The listing builds one solid part. Answer for the finished solid, in the listing's coordinates (mm). Face numbers are marked on the shaded views. A direction names the side the tool comes from. Coordinates: 2 decimals unless noted, no trailing zeros. Write each loop counter-clockwise with the first axis right and the second up, starting at its lowest first coordinate (ties: lowest second). Pieces come first, ordered by that corner, then holes. Notation, with made-up numbers: M 10.25,-30 L 50.25,-30 A21 ccw 50.25,-16 Z; hole C 38.25,-3.75 d5. An arc over 180 degrees is marked long. Answer as CSV lines item,"result". Start each with the question number.
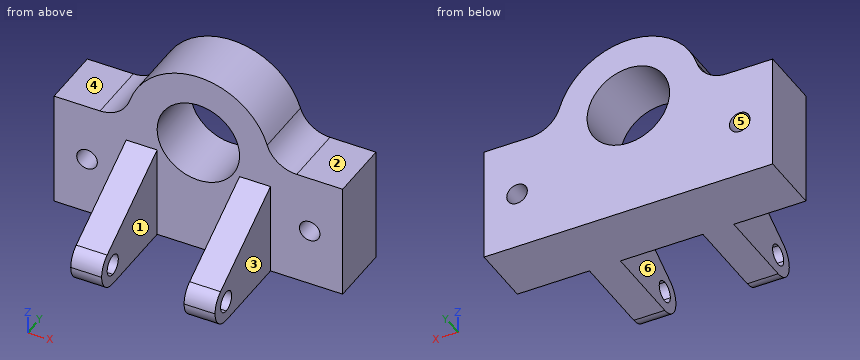
```python
from build123d import *

# Parameters (mm, degrees)
F1_DEPTH = 30
F2_R     = 15
F3_R     = 5
F4_DEPTH = 72
F6_DEPTH = 60
F8_DEPTH = 51.3


with BuildPart() as f1:
    # F0 (on Front) → F1 (new body)
    with BuildSketch(Plane.XZ):
        with BuildLine():
            Line((70, -28), (70, 28))
            Line((70, 28), (35, 28))
            ThreePointArc((35, 28), (0, -7), (-35, 28))
            Line((-35, 28), (-70, 28))
            Line((-70, 28), (-70, -28))
            Line((-70, -28), (70, -28))
        make_face()
        with BuildLine():
            ThreePointArc((-35, 28), (0, -7), (35, 28))
            Line((35, 28), (20, 28))
            ThreePointArc((20, 28), (0, 8), (-20, 28))
            Line((-20, 28), (-35, 28))
        make_face()
        with BuildLine():
            Line((20, 28), (35, 28))
            ThreePointArc((35, 28), (0, 63), (-35, 28))
            Line((-35, 28), (-20, 28))
            ThreePointArc((-20, 28), (0, 48), (20, 28))
        make_face()
    extrude(amount=F1_DEPTH)

    # F2
    f2_edges = [f1.edges().sort_by_distance(p)[0] for p in [
        (-35, -15, 28),
        (35, -15, 28),
    ]]
    fillet(f2_edges, radius=F2_R)

    # F3 (on face) → F4 (cut)
    with BuildSketch(Plane.XZ.offset(30)):
        with BuildLine():
            ThreePointArc((-49, 0), (-54, 5), (-59, 0))
            ThreePointArc((-59, 0), (-54, -5), (-49, 0))
        make_face()
        with Locations((54, 0)):
            Circle(F3_R)
    extrude(amount=-F4_DEPTH, mode=Mode.SUBTRACT)

    # F5 (on face) → F6 (join)
    with BuildSketch(Plane.XZ.offset(30)):
        Polygon((-35, 17), (-35, 0), (-35, -28), (-20, -28), (-20, 17), align=None)
    extrude(amount=F6_DEPTH)

    # F7 (on face) → F8 (cut)
    with BuildSketch(Plane(origin=(-35, 0, 0), x_dir=(0, -1, 0), z_dir=(-1, 0, 0))):
        with BuildLine():
            Line((90, 17), (30, 17))
            Line((30, 17), (75.0515173064, -9.369694507))
            ThreePointArc((75.0515173064, -9.369694507), (78.6751130559, -13.0258253481), (80, -18))
            ThreePointArc((80, -18), (77.0710678119, -25.0710678119), (70, -28))
            Line((70, -28), (90, -28))
            Line((90, -28), (90, 17))
        make_face()
        with BuildLine():
            ThreePointArc((70, -13), (65, -18), (70, -23))
            Line((70, -23), (70, -13))
        make_face()
        with BuildLine():
            Line((70, -13), (70, -23))
            ThreePointArc((70, -23), (73.5355339059, -21.5355339059), (75, -18))
            ThreePointArc((75, -18), (73.5355339059, -14.4644660941), (70, -13))
        make_face()
    extrude(amount=-F8_DEPTH, mode=Mode.SUBTRACT)

    # F9: F1 across plane


with BuildPart() as f1_1:
    add(f1.part)
    add(f1.part.mirror(Plane.YZ))


solid = f1_1.part
```
1) The part is cut by section A-A (x = -54). Determine the outline of the cut face in (y, z).
2) The part is cut by section C-C (z = 11). Determine the outline of the cut face in (x, y), then the cut area to 3 significant figures.
3) Which of the six approach directions +Z, -Z, +X, -X, +Y, -Y give full straight-line access (tool end or side, diameter ignored) to the marked faces 1, 2 and 3?
4) Find the intervals of material crossed by line 1 (Z direction, x = 54, y = -15); line 2 (X direction, y = -47.5, z = -17.5); line 3 (Z direction, x = 0, y = -16), in increasing order. Write a range as from..to.
5) Each of these flat-tipped pins is pushed along its axis until it touches: P1, Ø3, axis at x = 23.5, z = -10.5, coming from the +Y side; P2, Ø11, axis at x = 59.5, y = -17, coming from the +Z side; P3, Ø2, axis at x = -15.5, y = -14.5, coming from the +Z side; P4, Ø16, axis at x = 54, z = 0, coming from the -Y side. Where does it stop, or does it pass through?
6) For a pull along Z with two mould halves and no side action, classify the marked faces 4, 5 and 6 as +Z half, -Z half, draft (parallel to the pull), parting line (faces both ways), or undercut.
7) The part is cut by section B-B (y = -46). Determine the outline of the cut face in (x, z), then the cut area to 3 significant figures.
8) The part is cut by section D-D (y = -8.5). Determine the outline of the cut face in (x, z), then the cut area to 3 significant figures.
Completed:
1,outline,"M -30,-28 L 0,-28 L 0,-5 L -30,-5 Z; M -30,5 L 0,5 L 0,28 L -30,28 Z"
2,outline,"M -70,-30 L -35,-30 L -35,-40.25 L -20,-40.25 L -20,-30 L -10.54,-30 L -10.54,0 L -70,0 Z; M 10.54,-30 L 20,-30 L 20,-40.25 L 35,-40.25 L 35,-30 L 70,-30 L 70,0 L 10.54,0 Z"
2,area,"3,880 mm²"
3,face 1,"+Z, -Z, -Y"
3,face 2,"+Z, +X, +Y, -Y"
3,face 3,"+Z, -Z, +X, -Y"
4,line 1,"-28..-5, 5..28"
4,line 2,"-35..-20, 20..35"
4,line 3,"-28..8, 48..63"
5,P1,"y = 0"
5,P2,"z = 28"
5,P3,"z = 59.86"
5,P4,"y = -30"
6,face 4,"+Z half"
6,face 5,"undercut"
6,face 6,"draft"
7,outline,"M -35,-28 L -20,-28 L -20,7.63 L -35,7.63 Z; M 20,-28 L 35,-28 L 35,7.63 L 20,7.63 Z"
7,area,"1,070 mm²"
8,outline,"M -70,-28 L 70,-28 L 70,28 L 47.7,28 A15 cw 33.39,38.5 A35 ccw -33.39,38.5 A15 cw -47.7,28 L -70,28 Z; hole C -54,0 d10; hole C 0,28 d40; hole C 54,0 d10"
8,area,"8,410 mm²"
